Part model, mm, in its own coordinate system. Face numbers are marked on the shaded views. A direction names the side the tool comes from. Give positions to 0.01 mm unless a question says otherwise; leave off trailing zeros. Order: outer loops, then holes, each group sorted by start corner. A loop starts at its lowest first (then second) coordinate and runs counter-clockwise, first axis right, second up. Notation, with made-up numbers: M 88.25,-31.5 L 135.25,-31.5 A31 ccw 135.25,-7.5 Z; hole C 74.25,35 d2. An arc over 180 degrees is marked long. Answer as a JSON object with one key per item and string values.
from build123d import *

# Parameters (mm, degrees)
F1_DEPTH  = 42.926
F2_R      = 15.9122903495
F3_DEPTH  = 217.932
F7_DEPTH  = 169.926
F9_DEPTH  = 157.734
F10_W     = 24.1890698671
F10_H     = 14.7000979632
F11_DEPTH = 166.116


with BuildPart() as f1:
    # F0 (on Front) → F1 (new body)
    with BuildSketch(Plane.XZ):
        Polygon((-3.4105652012, 57.7952452004), (-72.7279856801, 57.7952452004), (-73.0966925621, 3.0418548267), (-3.4105652012, 3.0418548267), align=None)
    extrude(amount=F1_DEPTH)


with BuildPart() as f3:
    # F2 (on Front) → F3 (new body)
    with BuildSketch(Plane.XZ):
        with Locations((-37.1474996209, -45.6278249621)):
            Circle(F2_R)
    extrude(amount=F3_DEPTH)


with BuildPart() as f7:
    # F6 (on face) → F7 (new body, symmetric)
    with BuildSketch(Plane.XZ):
        Polygon((76.4440670609, 28.0330423266), (25.8330944926, 28.0330423266), (25.8330944926, 5.3316229023), (76.4440670609, 5.3316229023), (76.4440670609, 13.3329443634), align=None)
    extrude(amount=F7_DEPTH, both=True)

    # F8 (on face) → F9 (join, symmetric)
    with BuildSketch(Plane.XZ):
        Polygon((76.4440670609, 5.3316229023), (25.8330944926, 5.3316229023), (-75.7609978318, 5.3316229023), (-75.7609978318, -6.763396319), (76.4440670609, -6.763396319), align=None)
    extrude(amount=F9_DEPTH, both=True)

    # F10 (on face) → F11 (join, symmetric)
    with BuildSketch(Plane.XZ):
        with Locations((88.5386019945, 20.682993345)):
            Rectangle(F10_W, F10_H)
    extrude(amount=F11_DEPTH, both=True)


solid = f7.part
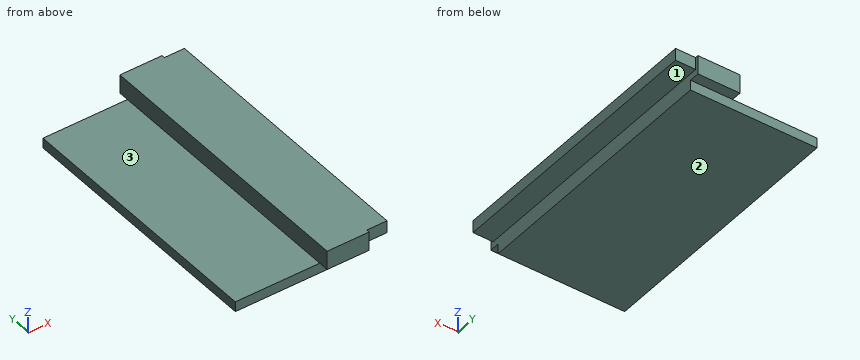
1. Which spindle directions (+Z, -Z, +X, -X, +Y, -Y) get a long thin tool onto all of the face, cutting with end or side? Do the marked faces 1, 2 and 3. Say none if no direction does.
Worked answers:
{"face 1": "-Z, +X, +Y, -Y", "face 2": "-Z, +X, -X, +Y, -Y", "face 3": "+Z, -X, +Y, -Y"}
2. Cut at A-A on x = 52. Give the cut face in (y, z).
Worked answers:
{"outline": "M -169.93,5.33 L -157.73,5.33 L -157.73,-6.76 L 157.73,-6.76 L 157.73,5.33 L 169.93,5.33 L 169.93,28.03 L -169.93,28.03 Z"}
3. Probe line 1 along Y through (x, z) = (44.5, 3.5); line 2 along Z through (x, y) = (-65.5, -132); line 3 along X through (y, z) = (-97.5, -3). List the from-to ranges inside material, lowest first.
Worked answers:
{"line 1": "y = -157.73 to 157.73", "line 2": "z = -6.76 to 5.33", "line 3": "x = -75.76 to 76.44"}
4. Pin check, flat tips, straight feed: P1, Ø9.5, axis at x = 9.5, z = 1.5, coming from the -Y side; P2, Ø12, axis at x = 90, y = -76.5, coming from the -Z side; P3, Ø12, axis at x = 92, z = 22.5, coming from the +Y side. Stop position of each tip, or through.
Worked answers:
{"P1": "stops at y = -157.73", "P2": "stops at z = 13.33", "P3": "stops at y = 166.12"}
5. Cut at D-D on x = -51. Give the cut face in (y, z), plus the area to 3 significant figures.
Worked answers:
{"outline": "M -157.73,-6.76 L 157.73,-6.76 L 157.73,5.33 L -157.73,5.33 Z", "area": "3,820 mm^2"}
6. Cut at C-C on z = -3. Give the cut face in (x, y), plus the area to 3 significant figures.
Worked answers:
{"outline": "M -75.76,-157.73 L 76.44,-157.73 L 76.44,157.73 L -75.76,157.73 Z", "area": "48,000 mm^2"}
7. Cut at B-B on y = -107. Give the cut face in (x, z).
Worked answers:
{"outline": "M -75.76,-6.76 L 76.44,-6.76 L 76.44,13.33 L 100.63,13.33 L 100.63,28.03 L 25.83,28.03 L 25.83,5.33 L -75.76,5.33 Z"}
